Autodesk Inventor part; units mm, degrees
ref_plane "YZ Plane" through (0, 0, 0) normal (1, 0, 0) x (0, 1, 0)
ref_plane "XZ Plane" through (0, 0, 0) normal (0, 1, 0) x (-1, 0, 0)
ref_plane "XY Plane" through (0, 0, 0) normal (0, 0, 1) x (1, 0, 0)
sketch "Sketch1" plane through (0, 0, 0) normal (0, 0, 1) x (1, 0, 0)
  line L0 (0, 0) -> (9.525, 0)
  line L1 (9.525, 0) -> (9.525, 6.35)
  line L2 (9.525, 6.35) -> (0, 6.35)
  line L3 (0, 6.35) -> (0, 0)
  dimension "d0" = 9.525
  dimension "d1" = 6.35
extrude "Extrusion1" add sketch "Sketch1" along normal blind 6.35
sketch "Sketch2" plane through (0, 6.35, 0) normal (0, 1, 0) x (1, 0, 0)
  point P0 (0, 0)
sketch "Sketch3" plane through (0, 6.35, 0) normal (0, 1, 0) x (1, 0, 0)
  line L0 (0, 0) -> (0, -6.35)
  line L1 (0, -6.35) -> (9.525, -6.35)
  line L2 (0, -3.175) -> (3.0988, -3.175)
  line L3 (3.0988, -3.175) -> (3.0988, -6.35)
  line L4 (3.0988, -6.35) -> (0, -6.35)
  line L5 (0, -6.35) -> (0, -3.175)
  dimension "d4" = 3.0988
extrude "Extrusion2" add sketch "Sketch3" along normal blind 3.175
sketch "Sketch4" plane through (0, 6.35, 0) normal (0, 1, 0) x (1, 0, 0)
  line L0 (9.525, 0) -> (9.525, -6.35)
  line L1 (0, -6.35) -> (9.525, -6.35)
  line L2 (9.525, -3.175) -> (6.4262, -3.175)
  line L3 (6.4262, -3.175) -> (6.4262, -6.35)
  line L4 (6.4262, -6.35) -> (9.525, -6.35)
  line L5 (9.525, -6.35) -> (9.525, -3.175)
  point P0 (0, 0)
  dimension "d7" = 3.0988
extrude "Extrusion3" add sketch "Sketch4" along normal blind 3.175
hole "Hole1" at (9.525, 7.9248, 4.7752) direction (-1, 0, 0) diameter 1.27 end through all
properties part number "HingePart2MK2"
Can you work these out from the model? Positions are in its coordinate system, mm. A direction names the side the tool comes from. Coordinates: 2 decimals unless noted, no trailing zeros. Order: outer loops, then holes, each group sorted by start corner. A loop starts at its lowest first (then second) coordinate and runs counter-clockwise, first axis right, second up.
1. I'm going to push flat-ended pins straight in: pin 1 (1.9 mm diameter, centred on x = 4.5, z = 2, fed in from +Y); pin 2 (1.5 mm diameter, centred on x = 2, y = 7.5, fed in from -Z) (3 decimals). Where does each tip first touch, or does it pass through?
2. If we section it at B-B (z = 4.5): Please give me the cut outline in (x, y) (3 decimals), then the cut area to 3 significant figures.
3. If we section it at D-D (x = 5.25): Please give me the cut outline in (y, z).
4. For faces 1 (the face through (8, 8, 3.175)), 2 (the face through (8, 9.525, 5)), which set-ups out of +Z, -Z, +X, -X, +Y, -Y let a thin tool reach every point of the face, with its end or its side?
5. Thinking about a two-plate mould opening in X: for faces 3 (the face through (9.525, 4, 3)), 4 (the face through (3.099, 9, 5)), 5 (the face through (2, 9.525, 5)), 6 (the face through (6.426, 9, 5)), which applies, +X half, -X half, draft (parallel to the pull), parting line (faces both ways), or undercut?
6. If we section it at C-C (x = 1): Please give me the cut outline in (y, z) (3 decimals), then the cut area to 3 significant figures.
7. I need wall thicknesses on line 1 (X direction, y = 8.5, z = 5.5) (3 decimals); line 2 (Y direction, x = 1.5, z = 3); line 3 (Y direction, x = 8.25, z = 5) (3 decimals). Which ranges of each line are inside material? Lowest first, please.
8. If we section it at A-A (y = 6.5): Please give me the cut outline in (x, z) (3 decimals).
Entries:
1. pin 1: stops at y = 6.35
1. pin 2: stops at z = 3.175
2. outline: (0, 0) - (9.525, 0) - (9.525, 7.353) - (6.426, 7.353) - (6.426, 6.35) - (3.099, 6.35) - (3.099, 7.353) - (0, 7.353) - close; (0, 8.497) - (3.099, 8.497) - (3.099, 9.525) - (0, 9.525) - close; (6.426, 8.497) - (9.525, 8.497) - (9.525, 9.525) - (6.426, 9.525) - close
2. area: 73.1 mm2
3. outline: (0, 0) - (6.35, 0) - (6.35, 6.35) - (0, 6.35) - close
4. face 1: -Z, +X, -X, +Y
4. face 2: +Z, -Z, +X, -X, +Y
5. face 3: +X half
5. face 4: undercut
5. face 5: draft
5. face 6: undercut
6. outline: (0, 0) - (6.35, 0) - (6.35, 3.175) - (9.525, 3.175) - (9.525, 6.35) - (0, 6.35) - close; hole circle Ø1.27 at (7.925, 4.775)
6. area: 49.1 mm2
7. line 1: x = 0 to 3.099, 6.426 to 9.525
7. line 2: y = 0 to 6.35
7. line 3: y = 0 to 7.331, 8.519 to 9.525
8. outline: (0, 3.175) - (3.099, 3.175) - (3.099, 6.35) - (0, 6.35) - close; (6.426, 3.175) - (9.525, 3.175) - (9.525, 6.35) - (6.426, 6.35) - close
